Here's how the part is built. I have some questions about the finished solid (model axes, mm). A direction names the side the tool comes from. Round coordinates to 2 decimals unless told otherwise and drop trailing zeros. Loops run counter-clockwise (first coordinate to the right, second up) from the corner with the lowest first, then second, coordinate; pieces in that order, holes last. Notation, with made-up numbers: (19, 26.5) - (77, 26.5) arc R29 cw to (77, 49.5) - close; hole circle Ø10 at (-7, 37.25). An arc over 180 degrees is marked (long way). Return JSON: item names as keys, results as strings. Group by question number.
```python
from build123d import *

# Parameters (mm, degrees)
SKETCH1_R           = 32.5
BOSS_EXTRUDE1_DEPTH = 10
CUT_EXTRUDE1_DEPTH  = 5
SKETCH3_R           = 2
CUT_EXTRUDE2_DEPTH  = 11
SKETCH4_R           = 20
BOSS_EXTRUDE2_DEPTH = 6
CUT_EXTRUDE3_DEPTH  = 17
SKETCH6_R           = 24
CUT_EXTRUDE5_DEPTH  = 7
CUT_EXTRUDE6_DEPTH  = 11
SKETCH8_W           = 45
SKETCH8_H           = 25
CUT_EXTRUDE7_DEPTH  = 8
FILLET1_R           = 3


with BuildPart() as part:
    # Sketch1 → Boss-Extrude1 (new body)
    with BuildSketch(Plane.XY):
        Circle(SKETCH1_R)
    extrude(amount=BOSS_EXTRUDE1_DEPTH)

    # Sketch2 → Cut-Extrude1 (cut)
    with BuildSketch(Plane.XY.offset(10)):
        Polygon((14.43375673, 0), (7.216878365, 12.5), (-7.216878365, 12.5), (-14.43375673, 0), (-7.216878365, -12.5), (7.216878365, -12.5), align=None)
    extrude(amount=-CUT_EXTRUDE1_DEPTH, mode=Mode.SUBTRACT)

    # Sketch3 → Cut-Extrude2 (cut, through all)
    with BuildSketch(Plane.XY.offset(10)):
        with Locations((0, 27.5)):
            Circle(SKETCH3_R)
        with Locations((19.445436483, 19.445436483)):
            Circle(SKETCH3_R)
        with Locations((27.5, 0)):
            Circle(SKETCH3_R)
        with Locations((19.445436483, -19.445436483)):
            Circle(SKETCH3_R)
        with Locations((0, -27.5)):
            Circle(SKETCH3_R)
        with Locations((-19.445436483, -19.445436483)):
            Circle(SKETCH3_R)
        with Locations((-27.5, 0)):
            Circle(SKETCH3_R)
        with Locations((-19.445436483, 19.445436483)):
            Circle(SKETCH3_R)
    extrude(amount=-CUT_EXTRUDE2_DEPTH, mode=Mode.SUBTRACT)

    # Sketch4 → Boss-Extrude2 (add)
    with BuildSketch(Plane(origin=(0, 0, 0), x_dir=(-1, 0, 0), z_dir=(0, 0, -1))):
        Circle(SKETCH4_R)
        Polygon((14.43375673, 0), (7.216878365, 12.5), (-7.216878365, 12.5), (-14.43375673, 0), (-7.216878365, -12.5), (7.216878365, -12.5), align=None, mode=Mode.SUBTRACT)
    extrude(amount=BOSS_EXTRUDE2_DEPTH)

    # Sketch5 → Cut-Extrude3 (cut, through all)
    with BuildSketch(Plane.XY.offset(10)):
        with BuildLine():
            Line((22.5, 23.452078799), (22.5, -23.452078799))
            ThreePointArc((22.5, -23.452078799), (32.5, 0), (22.5, 23.452078799))
        make_face()
        with BuildLine():
            Line((-22.5, 23.452078799), (-22.5, -23.452078799))
            ThreePointArc((-22.5, -23.452078799), (-32.5, 0), (-22.5, 23.452078799))
        make_face()
    extrude(amount=-CUT_EXTRUDE3_DEPTH, mode=Mode.SUBTRACT)

    # Sketch6 → Cut-Extrude5 (cut)
    with BuildSketch(Plane.XY.offset(10)):
        Circle(SKETCH6_R)
    extrude(amount=-CUT_EXTRUDE5_DEPTH, mode=Mode.SUBTRACT)

    # Sketch7 → Cut-Extrude6 (cut, through all)
    with BuildSketch(Plane(origin=(0, 0, 0), x_dir=(-1, 0, 0), z_dir=(0, 0, -1))):
        Polygon((14.43375673, 0), (7.216878365, 12.5), (-7.216878365, 12.5), (-14.43375673, 0), (-7.216878365, -12.5), (7.216878365, -12.5), align=None)
    extrude(amount=-CUT_EXTRUDE6_DEPTH, mode=Mode.SUBTRACT)

    # Sketch8 → Cut-Extrude7 (cut, through all)
    with BuildSketch(Plane.XY.offset(3)):
        Rectangle(SKETCH8_W, SKETCH8_H)
    extrude(amount=CUT_EXTRUDE7_DEPTH, mode=Mode.SUBTRACT)

    # Fillet1
    fillet1_edges = [part.edges().sort_by_distance(p)[0] for p in [
        (20, 0, 0),
    ]]
    fillet(fillet1_edges, radius=FILLET1_R)


solid = part.part
```
Q1. Imagine slicing it at D-D, the plane y = -27.5. List the corners of the cut face in (x, z) for me, and give its area (3 significant figures).
Q2. Please list where these lines run through material, in increasing order: line 1 (Y direction, x = 0, z = 8); line 2 (Z direction, x = -12, y = -24); line 3 (Z direction, x = 16.5, y = -1).
Q3. Imagine slicing it at B-B, the plane x = 0. List the corners of the cut face in (y, z) for me.
Q4. Will these pins go through, and if not, where does the flat tip stop? pin 1 Ø7 at (x, z) = (0, -0.5) entering from -Y; pin 2 Ø6.5 at (x, y) = (19.45, -19.45) entering from -Z; pin 3 Ø2.5 at (x, y) = (-19.45, 19.45) entering from +Z; pin 4 Ø2 at (x, z) = (21.5, 5.5) entering from +Y.
Q5. If we mould it in two halves opening along Y, with no side actions, what happens to faces 1 (the flat face through (-22.5, 0.3, 2.8)), 2 (the flat face through (-22, 12.5, 6)), 3 (the cylindrical face through (4.336, -19.524, -4.45)), 4 (the cylindrical face through (-17.54, 20.05, 5.07))? For each: +Y half, -Y half, draft (parallel to the pull), parting line (faces both ways), or undercut.
Q6. Imagine slicing it at A-A, the plane z = 4. List the corners of the cut face in (x, y) for me, and give its area (3 significant figures).
Q7. For faces 5 (the flat face through (0, 12.5, -2)), 6 (the cylindrical face through (0, -24, 7)), 7 (the flat face through (-22, -12.5, 6)), which set-ups out of +Z, -Z, +X, -X, +Y, -Y let a thin tool reach every point of the face, with its end or its side?
Q8. Imagine slicing it at C-C, the plane z = -4.5. List the corners of the cut face in (x, y) for me.
Output values:
{
 "1": {"outline": "(-17.32, 0) - (-2, 0) - (-2, 10) - (-17.32, 10) - close; (2, 0) - (17.32, 0) - (17.32, 10) - (2, 10) - close", "area": "306 mm^2"},
 "2": {"line 1": "y = -32.5 to -29.5, -25.5 to -24, 24 to 25.5, 29.5 to 32.5", "line 2": "z = 0 to 10", "line 3": "z = -6 to 3"},
 "3": {"outline": "(-32.5, 0) - (-29.5, 0) - (-29.5, 10) - (-32.5, 10) - close; (-25.5, 0) - (-23, 0) arc R3 cw to (-20, -3) - (-20, -6) - (-12.5, -6) - (-12.5, 3) - (-24, 3) - (-24, 10) - (-25.5, 10) - close; (12.5, -6) - (20, -6) - (20, -3) arc R3 cw to (23, 0) - (25.5, 0) - (25.5, 10) - (24, 10) - (24, 3) - (12.5, 3) - close; (29.5, 0) - (32.5, 0) - (32.5, 10) - (29.5, 10) - close"},
 "4": {"pin 1": "stops at y = -32.5", "pin 2": "stops at z = 0", "pin 3": "passes through", "pin 4": "stops at y = 25.22"},
 "5": {"face 1": "draft", "face 2": "undercut", "face 3": "parting line", "face 4": "undercut"},
 "6": {"outline": "(-22.5, -23.45) arc R32.5 ccw to (22.5, -23.45) - (22.5, -12.5) - (20.49, -12.5) arc R24 cw to (-20.49, -12.5) - (-22.5, -12.5) - close; (-22.5, 12.5) - (-20.49, 12.5) arc R24 cw to (20.49, 12.5) - (22.5, 12.5) - (22.5, 23.45) arc R32.5 ccw to (-22.5, 23.45) - close; hole circle Ø4 at (-19.45, -19.45); hole circle Ø4 at (-19.45, 19.45); hole circle Ø4 at (0, -27.5); hole circle Ø4 at (0, 27.5); hole circle Ø4 at (19.45, -19.45); hole circle Ø4 at (19.45, 19.45)", "area": "804 mm^2"},
 "7": {"face 5": "+Z, -Z", "face 6": "+Z", "face 7": "+Z, +X, -X"},
 "8": {"outline": "circle Ø40 at (0, 0); hole (-14.43, 0) - (-7.22, -12.5) - (7.22, -12.5) - (14.43, 0) - (7.22, 12.5) - (-7.22, 12.5) - close"}
}
